```python
from build123d import *
from OCP.BRepFilletAPI import BRepFilletAPI_MakeChamfer

# Parameters (mm, degrees)
SKETCH_1_W        = 30
SKETCH_1_H        = 3
DRAFT_1_ANGLE     = 1.15
CHAMFER_1_SIZE    = 0.5
CHAMFER_1_SIZE2   = 0.490259275
CHAMFER_1_SIZE2_2 = 0.510345395


with BuildPart() as part:
    # 草图1 → 旋转1 (revolve)
    with BuildSketch(Plane.XY, mode=Mode.PRIVATE) as revolve_1_sk:
        with Locations((15, 1.5)):
            Rectangle(SKETCH_1_W, SKETCH_1_H)
    revolve(revolve_1_sk.sketch.rotate(Axis((30, 0, 0), (-1, 0, 0)), 90), axis=Axis((30, 0, 0), (-1, 0, 0)))

    # 拔模1
    draft_1_faces = [part.faces().sort_by_distance(p)[0] for p in [
        (15, 0, 3),
    ]]
    draft(draft_1_faces, Plane(origin=(0, 0, 0), x_dir=(0, 0, -1), z_dir=(-1, 0, 0)), DRAFT_1_ANGLE)

    # 倒角1: one chamfer whose edges measure the first distance from different faces: ONE call of the kernel's chamfer builder (chamfer() names one face for all edges)
    chamfer_1_edges_1 = [part.edges().sort_by_distance(p)[0] for p in [
        (30, 0, 3.602219463),
    ]]
    chamfer_1_side_1 = [part.faces().sort_by_distance(p)[0] for p in [
        (15, 0, 3.301109732),
    ]]
    chamfer_1_edges_2 = [part.edges().sort_by_distance(p)[0] for p in [
        (0, 0, 3),
    ]]
    chamfer_1_side_2 = [part.faces().sort_by_distance(p)[0] for p in [
        (0, 0, 0),
    ]]
    chamfer_1 = BRepFilletAPI_MakeChamfer(part.part.solid().wrapped)
    for e in chamfer_1_edges_1:
        chamfer_1.Add(CHAMFER_1_SIZE, CHAMFER_1_SIZE2, e.wrapped, chamfer_1_side_1[0].wrapped)  # the first distance lies on this face
    for e in chamfer_1_edges_2:
        chamfer_1.Add(CHAMFER_1_SIZE, CHAMFER_1_SIZE2_2, e.wrapped, chamfer_1_side_2[0].wrapped)  # the first distance lies on this face
    add(Compound.cast(chamfer_1.Shape()), mode=Mode.REPLACE)


solid = part.part
```
Could you check a few things on this model? Use its own coordinates, in mm. A direction names the side the tool comes from. Round coordinates to 2 decimals unless told otherwise and drop trailing zeros. Loops run counter-clockwise (first coordinate to the right, second up) from the corner with the lowest first, then second, coordinate; pieces in that order, holes last. Notation, with made-up numbers: M 24.25,62.5 L 75.25,62.5 A26 cw 75.25,80.5 Z; hole C 28.25,82 d9. An arc over 180 degrees is marked long. Answer as CSV lines item,"result".
1) For pin 1 Ø2 at (x, y) = (13.5, 0.5) entering from -Z; pin 2 Ø1.5 at (x, z) = (22, 0.5) entering from +Y; pin 3 Ø1 at (x, z) = (10, -1) entering from +Y, each with a flat end and sliding along its axis, tell me the tip position at first contact or that it passes through.
From the geometry:
pin 1,"z = -3.29"
pin 2,"y = 3.45"
pin 3,"y = 3.16"
2) Imagine slicing it at A-A on z = 0. List the corners of the cut face in (x, y) for me.
From the geometry:
outline,"M 0,-2.5 L 0.51,-3.01 L 29.5,-3.59 L 30,-3.11 L 30,3.11 L 29.5,3.59 L 0.51,3.01 L 0,2.5 Z"
3) If I drill on probe 1 along Y at (x, z) = (22, 0.25); probe 2 along Y at (x, z) = (4.75, 2.5); probe 3 along Z at (x, y) = (17, -0.5), over which ranges is the centre line in solid material (lowest first)?
From the geometry:
probe 1,"-3.43 to 3.43"
probe 2,"-1.83 to 1.83"
probe 3,"-3.3 to 3.3"
4) Which directions (+Z, -Z, +X, -X, +Y, -Y) give clear straight access to the entire face, cutting with the end or side of a thin tool? Please do faces 1 (the conical face through (15.208, -0.993, -3.153)), 2 (the flat face through (0, 0, 0)).
From the geometry:
face 1,"-X"
face 2,"+Z, -Z, -X, +Y, -Y"
5) Imagine slicing it at B-B on x = 9.5. List the corners of the cut face in (y, z) for me, and give its area (3 significant figures).
From the geometry:
outline,"C 0,0 d6.38"
area,"32.0 mm^2"
